Design review of the part built by this model. Coordinates are the model's own, in mm. A direction names the side the tool comes from. Round coordinates to 2 decimals unless told otherwise and drop trailing zeros. Order: outer loops, then holes, each group sorted by start corner. A loop starts at its lowest first (then second) coordinate and runs counter-clockwise, first axis right, second up. Notation, with made-up numbers: (-28, 46.25) - (-23, 46.25) arc R9 cw to (-23, 63.25) - close; hole circle Ø4 at (55.5, -38). An arc over 180 degrees is marked (long way). Write item = value, one per line.
from build123d import *

# Parameters (mm, degrees)
BOSS_EXTRU_1_DEPTH      = 3.81
ESQUISSE2_R             = 7.62
BOSS_EXTRU_2_DEPTH      = 1.27
ESQUISSE3_R             = 4.826
BOSS_EXTRU_3_DEPTH      = 1.27
ESQUISSE4_R             = 5.334
BOSS_EXTRU_4_DEPTH      = 1.27
ESQUISSE5_R             = 4
ENL_V_MAT_EXTRU_1_DEPTH = 16.709032434


with BuildPart() as part:
    # Esquisse1 → Boss.-Extru.1 (new, symmetric)
    with BuildSketch(Plane.XY):
        Polygon((7.332348419, 0), (3.666174209, 6.35), (-3.666174209, 6.35), (-7.332348419, 0), (-3.666174209, -6.35), (3.666174209, -6.35), align=None)
    extrude(amount=BOSS_EXTRU_1_DEPTH, both=True)

    # Esquisse2 → Boss.-Extru.2 (add)
    with BuildSketch(Plane(origin=(0, 0, -3.81), x_dir=(-1, 0, 0), z_dir=(0, 0, -1))):
        Circle(ESQUISSE2_R)
    extrude(amount=BOSS_EXTRU_2_DEPTH)

    # Esquisse3 → Boss.-Extru.3 (add)
    with BuildSketch(Plane.XY.offset(3.81)):
        Circle(ESQUISSE3_R)
    extrude(amount=BOSS_EXTRU_3_DEPTH)

    # Esquisse4 → Boss.-Extru.4 (add)
    with BuildSketch(Plane.XY.offset(5.08)):
        Circle(ESQUISSE4_R)
    extrude(amount=BOSS_EXTRU_4_DEPTH)

    # Esquisse5 → Enlèv. mat.-Extru.1 (cut, through all)
    with BuildSketch(Plane(origin=(0, 0, -5.08), x_dir=(-1, 0, 0), z_dir=(0, 0, -1))):
        Circle(ESQUISSE5_R)
    extrude(amount=-ENL_V_MAT_EXTRU_1_DEPTH, mode=Mode.SUBTRACT)


solid = part.part
1) We need section C-C on y = -0.25. Write out the cut boundary in (x, z).
Findings:
outline = (-7.62, -5.08) - (-3.99, -5.08) - (-3.99, 6.35) - (-5.33, 6.35) - (-5.33, 5.08) - (-4.82, 5.08) - (-4.82, 3.81) - (-7.19, 3.81) - (-7.19, -3.81) - (-7.62, -3.81) - close; (3.99, -5.08) - (7.62, -5.08) - (7.62, -3.81) - (7.19, -3.81) - (7.19, 3.81) - (4.82, 3.81) - (4.82, 5.08) - (5.33, 5.08) - (5.33, 6.35) - (3.99, 6.35) - close
2) The part is to be moulded in two halves that separate along Z. For faces 1 (the flat face through (-5.525, -3.131, 0.053)), 2 (the cylindrical face through (-3.83, -2.937, 4.436)), 3 (the flat face through (-2, -4, 6.35)), say which applies: released by +Z, released by -Z, zero draft, split by the parting line, or undercut.
Findings:
face_1 = zero draft
face_2 = undercut
face_3 = released by +Z
3) To check wall thickness, follow L1, parallel to Y at x = 0, z = 4; L2, parallel to Y at x = 0, z = 0; L3, parallel to Z at x = -6.25, y = 0.25. State the ranges of each line that lie inside material, in increasing order. Write a range as from..to.
Findings:
L1 = -4.83..-4, 4..4.83
L2 = -6.35..-4, 4..6.35
L3 = -5.08..3.81
4) Clearance check with flat-ended pins moving along their axes: pin 1 Ø3 at (y, z) = (5, 0) entering from +X; pin 2 Ø6 at (x, z) = (0.5, 0) entering from -Y; pin 3 Ø1 at (x, z) = (-1, 5) entering from -Y. State where each tip first meets the part, or that it passes through.
Findings:
pin_1 = 5.31
pin_2 = -6.35
pin_3 = -5.31
5) We need section A-A on x = 0. Write out the cut boundary in (y, z).
Findings:
outline = (-7.62, -5.08) - (-4, -5.08) - (-4, 6.35) - (-5.33, 6.35) - (-5.33, 5.08) - (-4.83, 5.08) - (-4.83, 3.81) - (-6.35, 3.81) - (-6.35, -3.81) - (-7.62, -3.81) - close; (4, -5.08) - (7.62, -5.08) - (7.62, -3.81) - (6.35, -3.81) - (6.35, 3.81) - (4.83, 3.81) - (4.83, 5.08) - (5.33, 5.08) - (5.33, 6.35) - (4, 6.35) - close
6) We need section B-B on z = -0.25. Write out the cut boundary in (x, y), and give its area (3 significant figures).
Findings:
outline = (-7.33, 0) - (-3.67, -6.35) - (3.67, -6.35) - (7.33, 0) - (3.67, 6.35) - (-3.67, 6.35) - close; hole circle Ø8 at (0, 0)
area = 89.4 mm^2
7) We need section D-D on x = 6.25. Write out the cut boundary in (y, z).
Findings:
outline = (-4.36, -5.08) - (4.36, -5.08) - (4.36, -3.81) - (1.87, -3.81) - (1.87, 3.81) - (-1.87, 3.81) - (-1.87, -3.81) - (-4.36, -3.81) - close
8) For faces 4 (the flat face through (5.474, -3.219, 0.053)), 5 (the cylindrical face through (2.461, -4.732, 5.706)), 6 (the flat face through (5.525, 3.131, 0.053)), 7 (the flat face through (-5.474, 3.219, 0.053)), 8 (the flat face through (0, 6.35, 0)), list the 3-axis set-ups (+Z, -Z, +X, -X, +Y, -Y) from which the entire face can be reached by the end or side of a thin tool; tool diameter is ignored.
Findings:
face_4 = +Z, +X, -Y
face_5 = +Z
face_6 = +Z, +X, +Y
face_7 = +Z, -X, +Y
face_8 = +Z, +X, -X, +Y
